Autodesk Inventor part; units mm, degrees
ref_plane "РабПлоскость1" through (17.5, 36.1, 84) normal (0, 1, 0) x (1, 0, 0)
ref_plane "YZ Plane" through (0, 0, 0) normal (1, 0, 0) x (0, 1, 0)
ref_plane "XZ Plane" through (0, 0, 0) normal (0, 1, 0) x (-1, 0, 0)
sketch "Эскиз1" plane through (0, 0, 0) normal (0, 1, 0) x (-1, 0, 0)
  arc A0 (6.0208, -6) -> (6.0208, 6) centre (0, 0) ccw
  line L0 (6.0208, -6) -> (-6.0208, -6)
  arc A1 (-6.0208, 6) -> (-6.0208, -6) centre (0, 0) ccw
  line L1 (6.0208, 6) -> (-6.0208, 6)
  line L2 (17.5, 37) -> (-17.5, 37)
  line L3 (-17.5, 37) -> (-17.5, 0)
  arc A2 (-17.5, 0) -> (17.5, 0) centre (0, 0) ccw
  line L4 (17.5, 0) -> (17.5, 37)
  line L5 (17.5, 0) -> (17.5, 57)
  line L6 (-17.5, 37) -> (17.5, 37)
  line L7 (17.5, 37) -> (17.5, 57)
  line L8 (17.5, 57) -> (-17.5, 57)
  line L9 (-17.5, 57) -> (-17.5, 37)
extrude "Выдавливание1" add sketch "Эскиз1" along normal blind 27
sketch "Эскиз2" plane through (-17.5, 0, 57) normal (0, 0, 1) x (1, 0, 0)
  line L0 (0, 0) -> (35, 0)
  line L1 (35, 0) -> (35, 72.2)
  line L2 (35, 72.2) -> (0, 72.2)
  line L3 (0, 72.2) -> (0, 0)
  point P0 (17.5, 0)
  dimension "d2" = 72.2
extrude "Выдавливание2" add sketch "Эскиз2" along normal blind 27
ref_plane "РабПлоскость1" through (17.5, 36.1, 84) normal (0, 1, 0) x (1, 0, 0)
mirror "Зеркальное отражение1" about plane through (17.5, 36.1, 84) normal (0, 1, 0) of "Выдавливание1"
sketch "Эскиз3" plane through (17.5, 0, 0) normal (1, 0, 0) x (0, 0, -1)
  line L0 (-57, 45.2) -> (-57, 27)
  line L1 (-57, 36.1) -> (-42, 36.1)
  circle A0 centre (-42, 36.1) radius 18
  point P0 (0, 0)
  dimension "d5" = 15
  dimension "d6" = 36
extrude "Выдавливание3" cut sketch "Эскиз3" against normal blind 93.5
chamfer "Фаска2" distance 8 angle 45 8 edges at (0, 27, 26.4697) (0, 45.2, 26.4697) (-17.5, 27, 13.2349) (0, 27, -17.5) (17.5, 27, 13.2349) (-17.5, 45.2, 13.2349) (0, 45.2, -17.5) (17.5, 45.2, 13.2349)
properties part number "joint_2_part1"
Build history of the part. All positions in model axes, mm. A direction names the side the tool comes from. Round coordinates to 2 decimals unless told otherwise and drop trailing zeros. Order: outer loops, then holes, each group sorted by start corner. A loop starts at its lowest first (then second) coordinate and runs counter-clockwise, first axis right, second up. Notation, with made-up numbers: (46.25, 30) -> (68.25, 30) arc R33 cw to (68.25, 69) -> close; hole circle Ø2 at (13, 41). An arc over 180 degrees is marked (long way). Answer in a Markdown table with one row per item.
1) Pin check, flat tips, straight feed: P1, Ø9.5, axis at x = -0.5, y = 11, coming from the -Z side; P2, Ø9.5, axis at x = 2.5, z = -0.5, coming from the -Y side. Stop position of each tip, or through.
Values:
| item | result |
|---|---|
| P1 | z = -17.5 |
| P2 | through |
2) Band-saw the part on B-B on x = 0. Give the cut face in (y, z), and give its area (3 significant figures).
Values:
| item | result |
|---|---|
| outline | (0, -17.5) -> (19, -17.5) -> (27, -9.5) -> (27, -6) -> (0, -6) -> close; (0, 6) -> (27, 6) -> (27, 18.47) -> (21.17, 31.95) arc R18 cw (long way) to (51.03, 31.95) -> (45.2, 18.47) -> (45.2, 6) -> (72.2, 6) -> (72.2, 84) -> (0, 84) -> close; (45.2, -9.5) -> (53.2, -17.5) -> (72.2, -17.5) -> (72.2, -6) -> (45.2, -6) -> close |
| area | 4,790 mm2 |
3) Wall check: L1, parallel to Y at x = 2, z = 42; L2, parallel to X at y = 60.5, z = 0; L3, parallel to Z at x = 10, y = 36. Give the ranges that are in metal, low to high.
Values:
| item | result |
|---|---|
| L1 | 0 to 18.1, 54.1 to 72.2 |
| L2 | -17.5 to -8.5, 8.5 to 17.5 |
| L3 | 60 to 84 |
4) Mould opens along X. For faces 5 (the conical face through (-0.2, 25.6, -10.9)), 6 (the flat face through (0, 72.2, 33)), 7 (the cylindrical face through (-8.5, 13.3, 0.1)) say: released by +X, released by -X, zero draft, split by the parting line, or undercut.
Values:
| item | result |
|---|---|
| face 5 | split by the parting line |
| face 6 | zero draft |
| face 7 | undercut |
5) Band-saw the part on C-C on y = 23. Give the cut face in (x, z), and give its area (3 significant figures).
Values:
| item | result |
|---|---|
| outline | (-17.5, 54.34) -> (17.5, 54.34) -> (17.5, 84) -> (-17.5, 84) -> close; (-13.5, 0) arc R13.5 ccw to (13.5, 0) -> (13.5, 27.71) -> (-13.5, 27.71) -> close; hole (-6.02, -6) -> (6.02, -6) arc R8.5 ccw to (6.02, 6) -> (-6.02, 6) arc R8.5 ccw to start |
| area | 1,890 mm2 |
6) Band-saw the part on A-A on z = 9. Give the cut face in (x, y), and give its area (3 significant figures).
Values:
| item | result |
|---|---|
| outline | (-17.5, 0) -> (17.5, 0) -> (17.5, 19) -> (9.5, 27) -> (-9.5, 27) -> (-17.5, 19) -> close; (-17.5, 53.2) -> (-9.5, 45.2) -> (9.5, 45.2) -> (17.5, 53.2) -> (17.5, 72.2) -> (-17.5, 72.2) -> close |
| area | 1,760 mm2 |
7) Which spindle directions (+Z, -Z, +X, -X, +Y, -Y) get a long thin tool onto all of the face, cutting with end or side? Do faces 1 (the flat face through (13.4, 49.1, 13.9)), 2 (the flat face through (0, 27, 8)), 3 (the cylindrical face through (8.5, 58.9, 0.1)), 4 (the cylindrical face through (0.385, 62.833, -17.496)). Say none if no direction does.
Values:
| item | result |
|---|---|
| face 1 | -Z, +X |
| face 2 | -Z, +X, -X |
| face 3 | +Y, -Y |
| face 4 | -Z, +Y, -Y |
8) Band-saw the part on D-D on z = 42. Give the cut face in (x, y).
Values:
| item | result |
|---|---|
| outline | (-17.5, 0) -> (17.5, 0) -> (17.5, 18.1) -> (-17.5, 18.1) -> close; (-17.5, 54.1) -> (17.5, 54.1) -> (17.5, 72.2) -> (-17.5, 72.2) -> close |
